Input: part model. Units: mm. Frame: model coordinates. Face numbers are marked on the shaded views. A direction names the side the tool comes from. Round coordinates to 2 decimals unless told otherwise and drop trailing zeros. Order: outer loops, then holes, each group sorted by start corner. A loop starts at its lowest first (then second) coordinate and runs counter-clockwise, first axis right, second up. Notation, with made-up numbers: (14.5, 61) - (58.5, 61) arc R35 ccw to (58.5, 98) - close; hole circle Ø9 at (33, 30.25). An arc over 180 degrees is marked (long way). One line per item, written item: value. Start each with the question number.
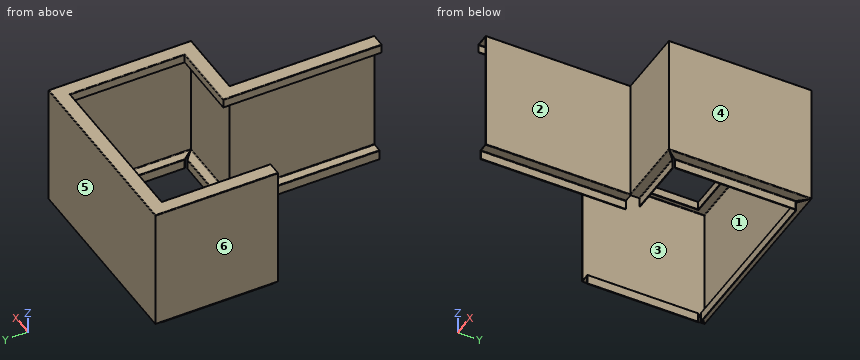
from build123d import *

# Parameters (mm, degrees)
F3_W     = 27
F3_H     = 27
F4_DEPTH = 40


with BuildPart() as f2:
    # F2: sweep along a path in F1
    with BuildLine(Plane.XY) as f2_path:
        Line((0, 0), (0, 346))
        Line((0, 346), (555, 346))
        Line((555, 346), (555, -57))
        Line((555, -57), (355, -57))
        Line((355, -57), (355, -464))
    # F0 (on Front) → F2 (sweep)
    with BuildSketch(Plane.XZ):
        with BuildLine():
            Line((38, 0), (2, 0))
            ThreePointArc((2, 0), (0.5857864376, -0.5857864376), (0, -2))
            Line((0, -2), (0, -348))
            ThreePointArc((0, -348), (0.5857864376, -349.4142135624), (2, -350))
            Line((2, -350), (25, -350))
            ThreePointArc((25, -350), (26.4142135624, -350.5857864376), (27, -352))
            Line((27, -352), (27, -376))
            Line((27, -376), (29, -376))
            Line((29, -376), (29, -350))
            ThreePointArc((29, -350), (28.4142135624, -348.5857864376), (27, -348))
            Line((27, -348), (4, -348))
            ThreePointArc((4, -348), (2.5857864376, -347.4142135624), (2, -346))
            Line((2, -346), (2, -4))
            ThreePointArc((2, -4), (2.5857864376, -2.5857864376), (4, -2))
            Line((4, -2), (36, -2))
            ThreePointArc((36, -2), (37.4142135624, -2.5857864376), (38, -4))
            Line((38, -4), (38, -25))
            Line((38, -25), (40, -25))
            Line((40, -25), (40, -2))
            ThreePointArc((40, -2), (39.4142135624, -0.5857864376), (38, 0))
        make_face()
    sweep(path=f2_path.line, transition=Transition.RIGHT)

    # F3 (on face) → F4 (cut)
    with BuildSketch(Plane.XY.offset(-348)):
        Polygon((2, 344), (29, 311.822653), (29, 317), (34.177347, 317), align=None)
        Polygon((526, 311.822653), (553, 344), (520.822653, 317), (526, 317), align=None)
        Polygon((520.822653, -28), (553, -55), (526, -22.822653), (526, -28), align=None)
        with Locations((339.5, -41.5)):
            Rectangle(F3_W, F3_H)
    extrude(amount=-F4_DEPTH, mode=Mode.SUBTRACT)


solid = f2.part
Item 1: Section query A-A on y = -317. Return loops of the section in (x, z), and give its area (3 significant figures).
Item 2: First-contact query: pin 1 Ø8 at (y, z) = (-129.5, -317.5) entering from +X; pin 2 Ø10 at (x, y) = (463, -46.5) entering from -Z; pin 3 Ø13.5 at (y, z) = (-41.5, -356) entering from -X. Flat tips, straight axial feed; report the tip coordinate or a pass-through.
Item 3: Section query B-B on z = -296. Return loops of the section in (x, y).
Item 4: Line query: L1, parallel to Z at x = 467.5, y = -49.5; L2, parallel to X at y = 292.5, z = -290.5; L3, parallel to Y at x = 396.5, z = -97. Output: solid intervals per line, ascending.
Item 5: Reachability of the marked faces 1 and 2 from +Z, -Z, +X, -X, +Y, -Y: full face, straight path, thin tool, end or side. Return the list, or none.
Item 6: Pull-direction query (X, two-part tool) for the marked faces 3, 4, 5 and 6; classes: released by +X, released by -X, zero draft, split by the parting line, or undercut.
Item 7: Section query C-C on x = 228. Return loops of the section in (y, z).
Geometry results:
1. outline: (315, -25) - (317, -25) - (317, -4) arc R2 cw to (319, -2) - (351, -2) arc R2 cw to (353, -4) - (353, -346) arc R2 cw to (351, -348) - (328, -348) arc R2 ccw to (326, -350) - (326, -376) - (328, -376) - (328, -352) arc R2 cw to (330, -350) - (353, -350) arc R2 ccw to (355, -348) - (355, -2) arc R2 ccw to (353, 0) - (317, 0) arc R2 ccw to (315, -2) - close
1. area: 928 mm^2
2. pin 1: stops at x = 355
2. pin 2: stops at z = -350
2. pin 3: stops at x = 353
3. outline: (0, 0) - (2, 0) - (2, 344) - (553, 344) - (553, -55) - (353, -55) - (353, -464) - (355, -464) - (355, -57) - (555, -57) - (555, 346) - (0, 346) - close
4. L1: z = -350 to -348, -2 to 0
4. L2: x = 0 to 2, 553 to 555
4. L3: y = -57 to -55, 344 to 346
5. face 1: none
5. face 2: +Z, -Z, +X, -Y
6. face 3: undercut
6. face 4: released by +X
6. face 5: zero draft
6. face 6: released by -X
7. outline: (306, -25) - (308, -25) - (308, -4) arc R2 cw to (310, -2) - (342, -2) arc R2 cw to (344, -4) - (344, -346) arc R2 cw to (342, -348) - (319, -348) arc R2 ccw to (317, -350) - (317, -376) - (319, -376) - (319, -352) arc R2 cw to (321, -350) - (344, -350) arc R2 ccw to (346, -348) - (346, -2) arc R2 ccw to (344, 0) - (308, 0) arc R2 ccw to (306, -2) - close
